```python
from build123d import *

# Parameters (mm, degrees)
SKETCH1_R           = 23.99268
SKETCH1_R_2         = 1.35
BOSS_EXTRUDE1_DEPTH = 2.5
CUT_EXTRUDE2_DEPTH  = 10


with BuildPart() as part:
    # Sketch1 → Boss-Extrude1 (new body)
    with BuildSketch(Plane(origin=(0, 0, 0), x_dir=(1, 0, 0), z_dir=(0, 1, 0))):
        Circle(SKETCH1_R)
        with Locations((0, 11.99634)):
            Circle(SKETCH1_R_2, mode=Mode.SUBTRACT)
        with Locations((10.389135192, -5.99817)):
            Circle(SKETCH1_R_2, mode=Mode.SUBTRACT)
        with Locations((-10.389135192, -5.99817)):
            Circle(SKETCH1_R_2, mode=Mode.SUBTRACT)
    extrude(amount=BOSS_EXTRUDE1_DEPTH)

    # Sketch3 → Cut-Extrude2 (cut)
    with BuildSketch(Plane(origin=(0, 2.5, 0), x_dir=(1, 0, 0), z_dir=(0, 1, 0))):
        with BuildLine():
            Line((5.735764364, 8.191520443), (8.603646545, 12.287280664))
            ThreePointArc((8.603646545, 12.287280664), (12.990381057, 7.5), (14.942920471, 1.307336141))
            Line((14.942920471, 1.307336141), (9.961946981, 0.871557427))
            ThreePointArc((9.961946981, 0.871557427), (8.660254038, 5), (5.735764364, 8.191520443))
        make_face()
        with BuildLine():
            Line((4.226182617, -9.06307787), (6.339273926, -13.594616806))
            ThreePointArc((6.339273926, -13.594616806), (0, -15), (-6.339273926, -13.594616806))
            Line((-6.339273926, -13.594616806), (-4.226182617, -9.06307787))
            ThreePointArc((-4.226182617, -9.06307787), (0, -10), (4.226182617, -9.06307787))
        make_face()
        with BuildLine():
            Line((-9.961946981, 0.871557427), (-14.942920471, 1.307336141))
            ThreePointArc((-14.942920471, 1.307336141), (-12.990381057, 7.5), (-8.603646545, 12.287280664))
            Line((-8.603646545, 12.287280664), (-5.735764364, 8.191520443))
            ThreePointArc((-5.735764364, 8.191520443), (-8.660254038, 5), (-9.961946981, 0.871557427))
        make_face()
    extrude(amount=-CUT_EXTRUDE2_DEPTH, mode=Mode.SUBTRACT)


solid = part.part
```
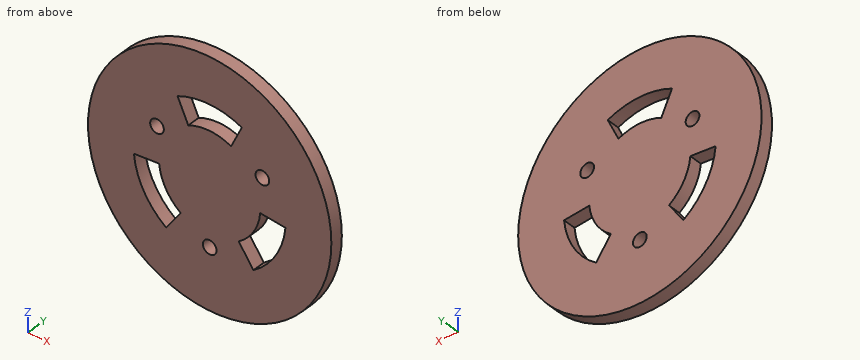
Here's how the part is built. I have some questions about the finished solid (model axes, mm). Give positions to 0.01 mm unless a question says otherwise; leave off trailing zeros. Write each loop counter-clockwise with the first axis right and the second up, starting at its lowest first coordinate (ties: lowest second). Pieces come first, ordered by that corner, then holes.
(1) Imagine slicing it at B-B, the plane y = 0.55. Write out the boundary of the cut face in (x, z).
Output values:
outline: circle Ø47.99 at (0, 0); hole (-14.94, -1.31) arc R15 ccw to (-8.6, -12.29) - (-5.74, -8.19) arc R10 cw to (-9.96, -0.87) - close; hole circle Ø2.7 at (-10.39, 6); hole (-6.34, 13.59) - (-4.23, 9.06) arc R10 cw to (4.23, 9.06) - (6.34, 13.59) arc R15 ccw to start; hole circle Ø2.7 at (0, -12); hole (5.74, -8.19) - (8.6, -12.29) arc R15 ccw to (14.94, -1.31) - (9.96, -0.87) arc R10 cw to start; hole circle Ø2.7 at (10.39, 6)
(2) Imagine slicing it at D-D, the plane x = 15.5. Write out the boundary of the cut face in (y, z), and give its area (3 significant figures).
Output values:
outline: (0, -18.31) - (2.5, -18.31) - (2.5, 18.31) - (0, 18.31) - close
area: 91.6 mm2
(3) Imagine slicing it at A-A, the plane x = 0. Write out the boundary of the cut face in (y, z), and give its area (3 significant figures).
Output values:
outline: (0, -23.99) - (2.5, -23.99) - (2.5, -13.35) - (0, -13.35) - close; (0, -10.65) - (2.5, -10.65) - (2.5, 10) - (0, 10) - close; (0, 15) - (2.5, 15) - (2.5, 23.99) - (0, 23.99) - close
area: 101 mm2
(4) Imagine slicing it at C-C, the plane z = -7. Write out the boundary of the cut face in (x, y).
Output values:
outline: (-22.95, 0) - (-13.27, 0) - (-13.27, 2.5) - (-22.95, 2.5) - close; (-7.14, 0) - (7.14, 0) - (7.14, 2.5) - (-7.14, 2.5) - close; (13.27, 0) - (22.95, 0) - (22.95, 2.5) - (13.27, 2.5) - close
(5) If I drill on L1, parallel to Z at x = 0, y = 1.55; L2, parallel to X at y = 1.15, z = -2.5; L3, parallel to X at y = 1.9, z = -11, over which ranges is the centre line in solid material (lowest first)?
Output values:
L1: z = -23.99 to -13.35, -10.65 to 10, 15 to 23.99
L2: x = -23.86 to -14.79, -9.68 to 9.68, 14.79 to 23.86
L3: x = -21.32 to -10.2, -7.7 to -0.91, 0.91 to 7.7, 10.2 to 21.32
